Read the model definition and answer for the solid it produces. Units are mm, in the model's axes. Coordinates: 2 decimals unless noted, no trailing zeros. Loops run counter-clockwise (first coordinate to the right, second up) from the corner with the lowest first, then second, coordinate; pieces in that order, holes last. Notation, with made-up numbers: M 69,0.5 L 93,0.5 A15 ccw 93,10.5 Z; hole C -17.75,-15 d6. An arc over 180 degrees is marked long. Use one line per item in the form item = value. Start each with the question number.
1. The part is cut by section A-A (y = 0). Give the vertices of the cut face in (x, z).
2. The part is cut by section B-B (z = -6). Give the vertices of the cut face in (x, y), plus the area to 3 significant figures.
3. Find the intervals of material crossed by probe 1 along X at (y, z) = (3, -6.25); probe 2 along X at (y, z) = (1.25, -4.25); probe 3 along X at (y, z) = (-1.25, -5.5), in increasing order. Write a range as [from, to].
4. For a pull along X with two mould halves and no side action, classify faces 1 (the cylindrical face through (4, 0, -4)), 2 (the cylindrical face through (-0.986, -7.493, 0.33)), 3 (the flat face through (-2, 0, 0)) as released by +X, released by -X, zero draft, split by the parting line, or undercut.
5. The part is cut by section D-D (z = 6). Give the vertices of the cut face in (x, y), plus the area to 3 significant figures.
6. The part is cut by section C-C (x = -1). Give the vertices of the cut face in (y, z), plus the area to 3 significant figures.
7. Flat-ended cylindrical pins translate along their axes: pin 1 (2 mm diameter, centred on x = 6, z = -6, fed in from +Y); pin 2 (5 mm diameter, centred on x = 3, z = -3, fed in from -Y); pin 3 (2 mm diameter, centred on x = -0.5, y = -1.5, fed in from -Z). Find the tip coordinate at first contact, or state that the pin passes through.
from build123d import *

# Parameters (mm, degrees)
F0_R     = 7.5
F1_DEPTH = 2
F3_R     = 1.5
F5_R     = 1.5


with BuildPart() as f1:
    # F0 (on Right) → F1 (new body)
    with BuildSketch(Plane.YZ):
        Circle(F0_R)
    extrude(amount=-F1_DEPTH)

    # F4: sweep along a path in F2
    with BuildLine(Plane.XZ) as f4_path:
        Line((0, 0), (2.5, 0))
        ThreePointArc((2.5, 0), (4.6213203436, -0.8786796564), (5.5, -3))
        Line((5.5, -3), (5.5, -6.5))
    # F3 (on Right) → F4 (sweep)
    with BuildSketch(Plane.YZ):
        Circle(F3_R)
    sweep(path=f4_path.line)

    # F5
    f5_edges = [f1.edges().sort_by_distance(p)[0] for p in [
        (5.5, -1.5, -6.5),
    ]]
    fillet(f5_edges, radius=F5_R)


solid = f1.part
Computed values:
q1.outline = M -2,-7.5 L 0,-7.5 L 0,-1.5 L 2.5,-1.5 A1.5 cw 4,-3 L 4,-5 A1.5 ccw 7,-5 L 7,-3 A4.5 ccw 2.5,1.5 L 0,1.5 L 0,7.5 L -2,7.5 Z
q2.outline = M -2,-4.5 L 0,-4.5 L 0,4.5 L -2,4.5 Z; C 5.5,0 d2.24
q2.area = 21.9 mm²
q3.probe_1 = [-2, 0]
q3.probe_2 = [-2, 0], [4.67, 6.33]
q3.probe_3 = [-2, 0], [4.84, 6.16]
q4.face_1 = undercut
q4.face_2 = zero draft
q4.face_3 = released by -X
q5.outline = M -2,-4.5 L 0,-4.5 L 0,4.5 L -2,4.5 Z
q5.area = 18.0 mm²
q6.outline = C 0,0 d15
q6.area = 177 mm²
q7.pin_1 = 1.5
q7.pin_2 = -1.5
q7.pin_3 = -7.48
